Source: three-view drawing plus pictorial views. Frame: mm from the lowest corner of the part. A direction names the side the tool comes from. Give positions to 0.01 mm unless a question says otherwise; leave off trailing zeros. Write each loop counter-clockwise with the first axis right and the second up, starting at its lowest first coordinate (ties: lowest second). Pieces come first, ordered by that corner, then holes. Notation, with made-up numbers: (68, -3.75) -> (119, -3.75) arc R27 ccw to (119, 33.25) -> close; hole circle Ø6 at (62, -30). An arc over 180 degrees is marked (long way). Use a Markdown table: item, result. Add a question column.
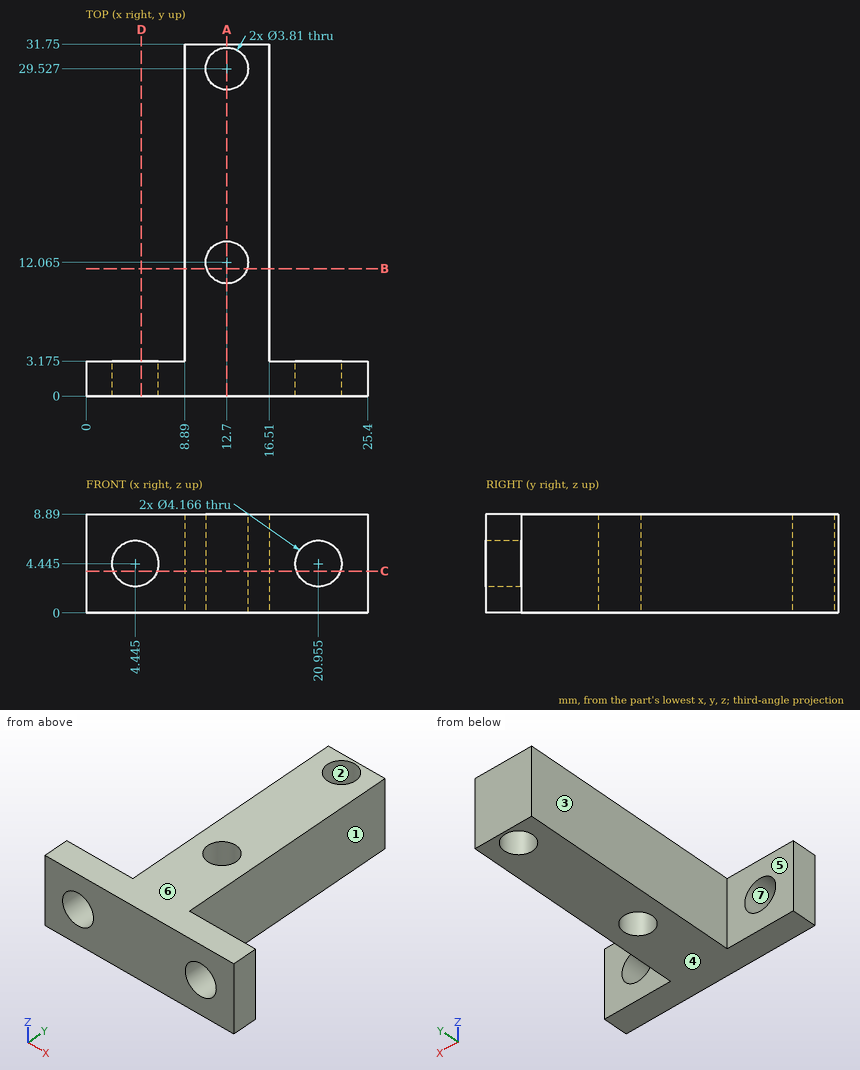
(1) Cut plane D-D on x = 5. Return the cut outline in (y, z) (1 decimal).
(2) First-contact query: pin 1 Ø3 at (y, z) = (16.5, 2.5) entering from -X; pin 2 Ø1 at (x, z) = (19, 1) entering from +Y (1 decimal); pin 3 Ø4.5 at (y, z) = (13, 3.5) entering from +X; pin 4 Ø2.5 at (x, z) = (4.445, 4.445) entering from +Y. Flat tips, straight axial feed; report the tip coordinate or a pass-through.
(3) Material intervals for L1, parallel to Y at x = 12.75, z = 8; L2, parallel to Y at x = 19.25, z = 6 (1 decimal); L3, parallel to X at y = 9.5, z = 6.5, sorted ascending.
(4) Access query for the marked faces 1, 2 and 3. Directions: +Z, -Z, +X, -X, +Y, -Y. A direction counts if a zero-diameter tool reaches every point of the face in a straight line with its end or side. Return the directions, or none.
(5) Mould query, pull axis Z, two halves, no side actions, for the marked faces 4, 5, 6 and 7. Classes: +Z half, -Z half, draft (parallel to the pull), parting line (faces both ways), or undercut.
(6) Cut plane A-A on x = 12.7. Return the cut outline in (y, z).
(7) Cut plane B-B on y = 11.5. Return the cut outline in (x, z).
(8) Cut plane C-C on z = 3.75. Count the separate pieces of the cut face and the enclosed holes in it, then the cut area to 3 significant figures.
Output:
| question | item | result |
|---|---|---|
| 1 | outline | (0, 0) -> (3.2, 0) -> (3.2, 2.4) -> (0, 2.4) -> close; (0, 6.5) -> (3.2, 6.5) -> (3.2, 8.9) -> (0, 8.9) -> close |
| 2 | pin 1 | x = 8.89 |
| 2 | pin 2 | y = 3.2 |
| 2 | pin 3 | x = 16.51 |
| 2 | pin 4 | through |
| 3 | L1 | 0 to 10.16, 13.97 to 27.62, 31.43 to 31.75 |
| 3 | L2 | 0 to 3.2 |
| 3 | L3 | 8.89 to 16.51 |
| 4 | face 1 | +Z, -Z, +X, +Y |
| 4 | face 2 | +Z, -Z |
| 4 | face 3 | +Z, -Z, -X, +Y |
| 5 | face 4 | -Z half |
| 5 | face 5 | draft |
| 5 | face 6 | +Z half |
| 5 | face 7 | undercut |
| 6 | outline | (0, 0) -> (10.16, 0) -> (10.16, 8.89) -> (0, 8.89) -> close; (13.97, 0) -> (27.62, 0) -> (27.62, 8.89) -> (13.97, 8.89) -> close; (31.43, 0) -> (31.75, 0) -> (31.75, 8.89) -> (31.43, 8.89) -> close |
| 7 | outline | (8.89, 0) -> (10.88, 0) -> (10.88, 8.89) -> (8.89, 8.89) -> close; (14.52, 0) -> (16.51, 0) -> (16.51, 8.89) -> (14.52, 8.89) -> close |
| 8 | separate pieces | 3 |
| 8 | enclosed holes | 2 |
| 8 | area | 251 mm^2 |
